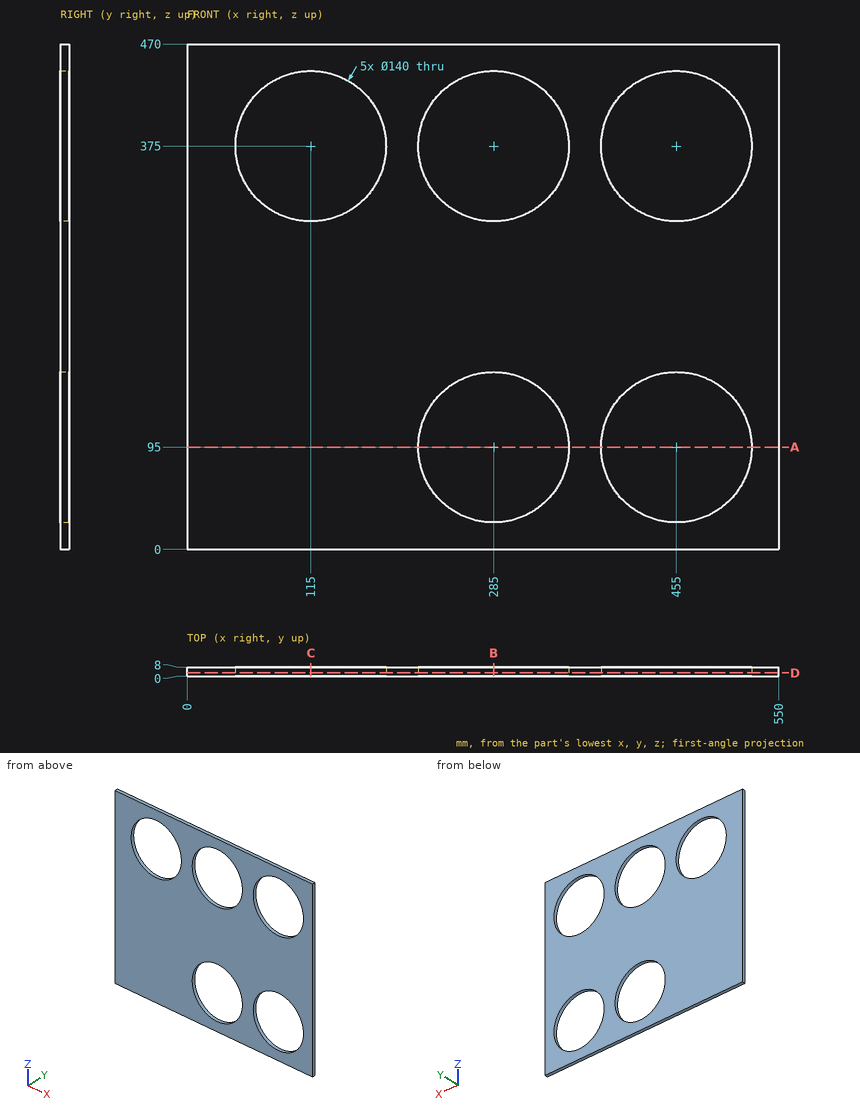
Verification items for this drawing (mm, ordinates from the low corner). Coordinates: 2 decimals unless noted, no trailing zeros. Write each loop counter-clockwise with the first axis right and the second up, starting at its lowest first coordinate (ties: lowest second). Pieces come first, ordered by that corner, then holes. Notation, with made-up numbers: (25, 2.25) -> (72, 2.25) arc R31 ccw to (72, 39.25) -> close; hole circle Ø10 at (82.25, 88). An arc over 180 degrees is marked (long way). One line per item, written item: value. Start each with the question number.
Q1. Thickness scan on L1, parallel to X at y = 1.5, z = 375; L2, parallel to X at y = 3.75, z = 95; L3, parallel to X at y = 6.25, z = 419.5. Record the ranges inside material, lowest first. Write a range as from..to.
Q2. Cross-section at B-B on x = 285. Enter the section's corners in (y, z), and give its area (3 significant figures).
Q3. Cross-section at C-C on x = 115. Enter the section's corners in (y, z), and give its area (3 significant figures).
Q4. Cross-section at A-A on z = 95. Enter the section's corners in (x, y), and give its area (3 significant figures).
Q5. Cross-section at D-D on y = 3. Enter the section's corners in (x, z), and give its area (3 significant figures).
Checked values:
1. L1: x = 0..45, 185..215, 355..385, 525..550
1. L2: x = 0..215, 355..385, 525..550
1. L3: x = 0..60.97, 169.03..230.97, 339.03..400.97, 509.03..550
2. outline: (0, 0) -> (8, 0) -> (8, 25) -> (0, 25) -> close; (0, 165) -> (8, 165) -> (8, 305) -> (0, 305) -> close; (0, 445) -> (8, 445) -> (8, 470) -> (0, 470) -> close
2. area: 1,520 mm²
3. outline: (0, 0) -> (8, 0) -> (8, 305) -> (0, 305) -> close; (0, 445) -> (8, 445) -> (8, 470) -> (0, 470) -> close
3. area: 2,640 mm²
4. outline: (0, 0) -> (215, 0) -> (215, 8) -> (0, 8) -> close; (355, 0) -> (385, 0) -> (385, 8) -> (355, 8) -> close; (525, 0) -> (550, 0) -> (550, 8) -> (525, 8) -> close
4. area: 2,160 mm²
5. outline: (0, 0) -> (550, 0) -> (550, 470) -> (0, 470) -> close; hole circle Ø140 at (115, 375); hole circle Ø140 at (285, 95); hole circle Ø140 at (285, 375); hole circle Ø140 at (455, 95); hole circle Ø140 at (455, 375)
5. area: 182,000 mm²
